The listing builds one solid part. Answer for the finished solid, in the listing's coordinates (mm). A direction names the side the tool comes from. Round coordinates to 2 decimals unless told otherwise and drop trailing zeros. Loops run counter-clockwise (first coordinate to the right, second up) from the corner with the lowest first, then second, coordinate; pieces in that order, holes last. Notation, with made-up numbers: (5, 15) -> (43, 15) arc R5 cw to (43, 19) -> close; hole circle Ø8 at (34, 57.5). An arc over 180 degrees is marked (long way). Use a Markdown table: item, result. Add a question column.
Q1. Section B-B on x = -5 is taken. Give the vertices of the cut face in (y, z).
Q2. Consider line 1 (Y direction, x = -5, z = 4); line 2 (Y direction, x = -1.25, z = 2); line 3 (Y direction, x = -6.75, z = 5.25). Determine where each line is inside the solid, lowest interval first.
Q3. Section A-A on z = 3.75 is taken. Give the vertices of the cut face in (x, y), then the cut area to 3 significant figures.
Q4. For a pull along X with two mould halves and no side action, classify faces 3 (the flat face through (-9, 60, 5)), 4 (the flat face through (-2.5, 30, 5)), 5 (the cylindrical face through (-5.26, -54.517, 5.07)), 6 (the flat face through (15, -6, 5)) as released by +X, released by -X, zero draft, split by the parting line, or undercut.
Q5. Section C-C on y = 28.5 is taken. Give the vertices of the cut face in (x, z).
Q6. Which of the six approach directions +Z, -Z, +X, -X, +Y, -Y give full straight-line access (tool end or side, diameter ignored) to faces 1 (the flat face through (0, 0, 5)), 2 (the cylindrical face through (4.74, -54.517, 5.07))?
Q7. Given pin 1 Ø2.5 at (x, z) = (0, 6.5) entering from +Y, flat-ended and moving along its own axis, determine where the tip first touches the part or whether it passes through.
Q8. Section D-D on y = -56.5 is taken. Give the vertices of the cut face in (x, z), then the cut area to 3 significant figures.
from build123d import *

# Parameters (mm, degrees)
ESBO_O1_W                = 30
ESBO_O1_H                = 140
RESSALTO_EXTRUS_O1_DEPTH = 10
CORTE_EXTRUS_O1_REACH    = 74.284
ESBO_O2_R                = 2
CORTE_EXTRUS_O2_REACH    = 78.811
ESBO_O3_W                = 10
ESBO_O3_H                = 10
CORTE_EXTRUS_O3_REACH    = 74.284
ESBO_O4_W                = 5
ESBO_O4_H                = 60


with BuildPart() as part:
    # Esboço1 → Ressalto-extrusão1 (new body)
    with BuildSketch(Plane.XY):
        Rectangle(ESBO_O1_W, ESBO_O1_H)
    extrude(amount=RESSALTO_EXTRUS_O1_DEPTH)

    # Esboço2 → Corte-extrusão1 (cut, up to next)
    with BuildSketch(Plane.XY.offset(10), mode=Mode.PRIVATE) as corte_extrus_o1_sk1:
        with Locations((-5, -56.5)):
            Circle(ESBO_O2_R)
    corte_extrus_o1_tool1 = extrude(corte_extrus_o1_sk1.sketch, amount=-CORTE_EXTRUS_O1_REACH, mode=Mode.PRIVATE) & part.part
    # Esboço2 → Corte-extrusão1 (cut, up to next)
    with BuildSketch(Plane.XY.offset(10), mode=Mode.PRIVATE) as corte_extrus_o1_sk2:
        with Locations((5, -56.5)):
            Circle(ESBO_O2_R)
    corte_extrus_o1_tool2 = extrude(corte_extrus_o1_sk2.sketch, amount=-CORTE_EXTRUS_O1_REACH, mode=Mode.PRIVATE) & part.part
    add(corte_extrus_o1_tool1.solids().sort_by_distance((-5, -56.5, 10))[0], mode=Mode.SUBTRACT)
    add(corte_extrus_o1_tool2.solids().sort_by_distance((5, -56.5, 10))[0], mode=Mode.SUBTRACT)

    # Esboço3 → Corte-extrusão2 (cut, up to next)
    with BuildSketch(Plane(origin=(15, 0, 0), x_dir=(0, 0, -1), z_dir=(1, 0, 0)), mode=Mode.PRIVATE) as corte_extrus_o2_sk1:
        with Locations((-5, 65)):
            Rectangle(ESBO_O3_W, ESBO_O3_H)
    corte_extrus_o2_tool1 = extrude(corte_extrus_o2_sk1.sketch, amount=-CORTE_EXTRUS_O2_REACH, mode=Mode.PRIVATE) & part.part
    add(corte_extrus_o2_tool1.solids().sort_by_distance((15, 65, 5))[0], mode=Mode.SUBTRACT)

    # Esboço4 → Corte-extrusão3 (cut, up to next)
    with BuildSketch(Plane.XY.offset(10), mode=Mode.PRIVATE) as corte_extrus_o3_sk1:
        with Locations((0, 30)):
            Rectangle(ESBO_O4_W, ESBO_O4_H)
    corte_extrus_o3_tool1 = extrude(corte_extrus_o3_sk1.sketch, amount=-CORTE_EXTRUS_O3_REACH, mode=Mode.PRIVATE) & part.part
    add(corte_extrus_o3_tool1.solids().sort_by_distance((0, 30, 10))[0], mode=Mode.SUBTRACT)


solid = part.part
Checked values:
| question | item | result |
|---|---|---|
| 1 | outline | (-70, 0) -> (-58.5, 0) -> (-58.5, 10) -> (-70, 10) -> close; (-54.5, 0) -> (60, 0) -> (60, 10) -> (-54.5, 10) -> close |
| 2 | line 1 | y = -70 to -58.5, -54.5 to 60 |
| 2 | line 2 | y = -70 to 0 |
| 2 | line 3 | y = -70 to -57.47, -55.53 to 60 |
| 3 | outline | (-15, -70) -> (15, -70) -> (15, 60) -> (2.5, 60) -> (2.5, 0) -> (-2.5, 0) -> (-2.5, 60) -> (-15, 60) -> close; hole circle Ø4 at (-5, -56.5); hole circle Ø4 at (5, -56.5) |
| 3 | area | 3,570 mm2 |
| 4 | face 3 | zero draft |
| 4 | face 4 | undercut |
| 4 | face 5 | undercut |
| 4 | face 6 | released by +X |
| 5 | outline | (-15, 0) -> (-2.5, 0) -> (-2.5, 10) -> (-15, 10) -> close; (2.5, 0) -> (15, 0) -> (15, 10) -> (2.5, 10) -> close |
| 6 | face 1 | +Z, -Z, +Y |
| 6 | face 2 | +Z, -Z |
| 7 | pin 1 | stops at y = 0 |
| 8 | outline | (-15, 0) -> (-7, 0) -> (-7, 10) -> (-15, 10) -> close; (-3, 0) -> (3, 0) -> (3, 10) -> (-3, 10) -> close; (7, 0) -> (15, 0) -> (15, 10) -> (7, 10) -> close |
| 8 | area | 220 mm2 |
